Could you check a few things on this model? Use its own coordinates, in mm. Round coordinates to 2 decimals unless told otherwise and drop trailing zeros. Loops run counter-clockwise (first coordinate to the right, second up) from the corner with the lowest first, then second, coordinate; pieces in that order, holes last. Notation, with made-up numbers: (43.5, -28) -> (74.5, -28) arc R21 ccw to (74.5, -7) -> close; hole circle Ø5 at (-1.75, 62). An arc over 180 degrees is marked (long way). One line per item, written item: value.
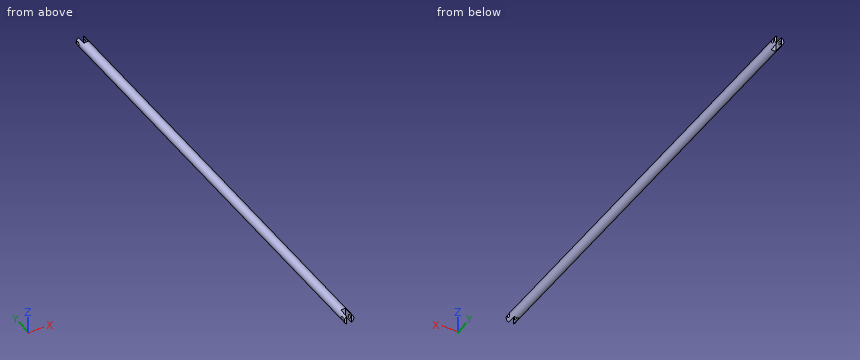
from build123d import *

# Parameters (mm, degrees)
F0_R      = 3.175
F1_DEPTH  = 298.45
F2_W      = 3.175
F2_H      = 13.081
F3_DEPTH  = 12.7
F4_R      = 1.27
F5_DEPTH  = 12.7
F6_DEPTH  = 19.05
F7_W      = 3.175
F7_H      = 12.7
F8_DEPTH  = 12.7
F9_R      = 1.27
F10_DEPTH = 12.7


with BuildPart() as f1:
    # F0 (on Front) → F1 (new body)
    with BuildSketch(Plane.XZ):
        Circle(F0_R)
    extrude(amount=F1_DEPTH)

    # F2 (on Top) → F3 (cut, symmetric)
    with BuildSketch(Plane.XY):
        Rectangle(F2_W, F2_H)
    extrude(amount=F3_DEPTH, both=True, mode=Mode.SUBTRACT)

    # F4 (on Right) → F5 (cut, symmetric)
    with BuildSketch(Plane.YZ):
        with Locations((-1.905, 0)):
            Circle(F4_R)
    extrude(amount=F5_DEPTH, both=True, mode=Mode.SUBTRACT)

    # F6 (add): a face of the model
    f6_faces = [f1.faces().sort_by_distance(p)[0] for p in [
        (0, -298.45, 0),
    ]]
    extrude(f6_faces, amount=F6_DEPTH)

    # F7 (on Top) → F8 (cut, symmetric)
    with BuildSketch(Plane.XY):
        with Locations((0, -316.9831931591)):
            Rectangle(F7_W, F7_H)
    extrude(amount=F8_DEPTH, both=True, mode=Mode.SUBTRACT)

    # F9 (on Right) → F10 (cut, symmetric)
    with BuildSketch(Plane.YZ):
        with Locations((-314.9411380291, 0)):
            Circle(F9_R)
    extrude(amount=F10_DEPTH, both=True, mode=Mode.SUBTRACT)


solid = f1.part
(1) If we section it at A-A, the plane z = 0: Please give me the cut outline in (x, y) (1 decimal), then the cut area to 3 significant figures.
Recorded:
outline: (-3.2, -317.5) -> (-1.6, -317.5) -> (-1.6, -316.2) -> (-3.2, -316.2) -> close; (-3.2, -313.7) -> (-1.6, -313.7) -> (-1.6, -310.6) -> (1.6, -310.6) -> (1.6, -313.7) -> (3.2, -313.7) -> (3.2, -3.2) -> (1.6, -3.2) -> (1.6, -6.5) -> (-1.6, -6.5) -> (-1.6, -3.2) -> (-3.2, -3.2) -> close; (-3.2, -0.6) -> (-1.6, -0.6) -> (-1.6, 0) -> (-3.2, 0) -> close; (1.6, -317.5) -> (3.2, -317.5) -> (3.2, -316.2) -> (1.6, -316.2) -> close; (1.6, -0.6) -> (3.2, -0.6) -> (3.2, 0) -> (1.6, 0) -> close
area: 1,960 mm²
(2) If I drill on L1, parallel to Y at x = 2.3, z = 0 (3 decimals); L2, parallel to Y at x = 2, z = 0.5; L3, parallel to Y at x = -1.5, z = 0.25, over which ranges is the centre line in solid material (lowest first)?
Recorded:
L1: -317.5 to -316.211, -313.671 to -3.175, -0.635 to 0
L2: -317.5 to -316.11, -313.77 to -3.07, -0.74 to 0
L3: -310.63 to -6.54
(3) If we section it at C-C, the plane y = -252.5: Please give me the cut outline in (x, z) (3 decimals).
Recorded:
outline: circle Ø6.35 at (0, 0)
(4) I'm going to push flat-ended pins straight in: pin 1 Ø2.5 at (x, z) = (0, 0.5) entering from -Y; pin 2 Ø3 at (y, z) = (-124, 2) entering from -X; pin 3 Ø3 at (x, y) = (-2.5, -212) entering from -Z. Where does each tip first touch, or does it pass through?
Recorded:
pin 1: y = -310.63
pin 2: x = -3.14
pin 3: z = -3.01
(5) If we section it at B-B, the plane x = 0: Please give me the cut outline in (y, z) (1 decimal).
Recorded:
outline: (-310.6, -3.2) -> (-6.5, -3.2) -> (-6.5, 3.2) -> (-310.6, 3.2) -> close
